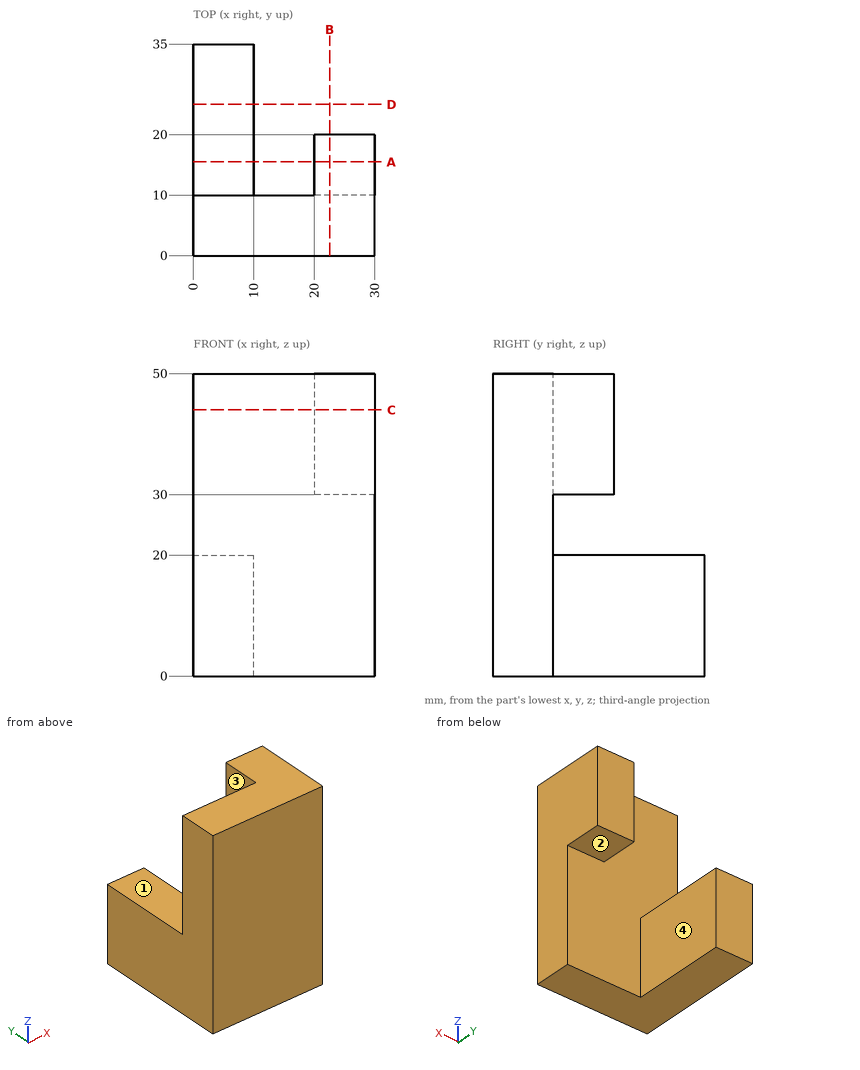
Drawing for the job (mm, zero at the part's lowest x, y, z). A direction names the side the tool comes from. Give positions to 0.01 mm unless a question says otherwise; leave off trailing zeros. Order: outer loops, then holes, each group sorted by start corner. A loop starts at its lowest first (then second) coordinate and runs counter-clockwise, first axis right, second up. Notation, with made-up numbers: M 63,8 L 80,8 A9 cw 80,17 Z; hole C 62,5 d4. An arc over 180 degrees is marked long. Put each result on its own line as item: value.
Item 1: Slice it at A-A, the plane y = 15.5. Write the cut outline in (x, z).
From the geometry:
outline: M 0,0 L 10,0 L 10,20 L 0,20 Z; M 20,30 L 30,30 L 30,50 L 20,50 Z
Item 2: Slice it at D-D, the plane y = 25. Write the cut outline in (x, z).
From the geometry:
outline: M 0,0 L 10,0 L 10,20 L 0,20 Z
Item 3: 3-axis set-ups, long thin cutter, end or side, ignore diameter. For the marked faces 1, 2, 3 and 4: which of +Z, -Z, +X, -X, +Y, -Y reach the whole face in a straight line?
From the geometry:
face 1: +Z, +X, -X, +Y
face 2: -Z, +X, -X, +Y
face 3: +Z, -Z, -X, +Y
face 4: +Z, -Z, +X, +Y
Item 4: Probe line 1 (X direction, y = 14, z = 38); line 2 (Y direction, x = 25, z = 12); line 3 (Y direction, x = 22.75, z = 32). List the from-to ranges inside material, lowest first. Write a range as [from, to].
From the geometry:
line 1: x = [20, 30]
line 2: y = [0, 10]
line 3: y = [0, 20]
Item 5: Flat gauge pins, fed straight in: pin 1 Ø11 at (x, z) = (27, 37) entering from +Y; pin 2 Ø5 at (x, y) = (3, 23) entering from +Z; pin 3 Ø5 at (y, z) = (13, 41.5) entering from -X. Where does each tip first touch, or does it go through?
From the geometry:
pin 1: stops at y = 20
pin 2: stops at z = 20
pin 3: stops at x = 20
Item 6: Slice it at B-B, the plane x = 22.5. Write the cut outline in (y, z).
From the geometry:
outline: M 0,0 L 10,0 L 10,30 L 20,30 L 20,50 L 0,50 Z
Item 7: Slice it at C-C, the plane z = 44. Write the cut outline in (x, y).
From the geometry:
outline: M 0,0 L 30,0 L 30,20 L 20,20 L 20,10 L 0,10 Z
